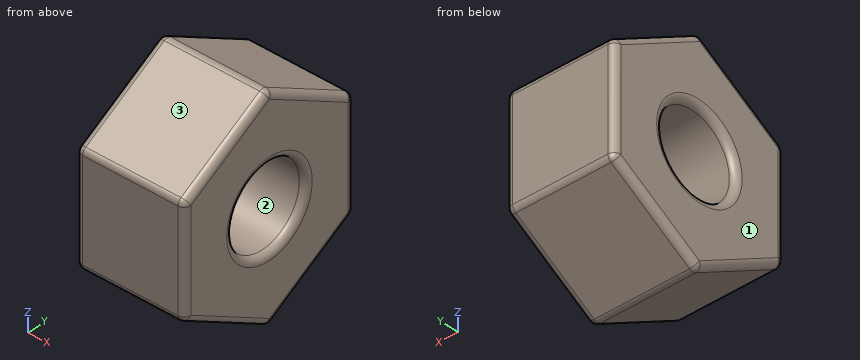
```python
from build123d import *

# Parameters (mm, degrees)
SKETCH1_R           = 3
BOSS_EXTRUDE1_DEPTH = 8
FILLET1_R           = 0.5


with BuildPart() as part:
    # Sketch1 → Boss-Extrude1 (new body)
    with BuildSketch(Plane.YZ):
        Polygon((-6.92820323, -4), (0, -8), (6.92820323, -4), (6.92820323, 4), (0, 8), (-6.92820323, 4), align=None)
        with Locations(Location((0, 0, 0), (0, 0, 270))):
            Circle(SKETCH1_R, mode=Mode.SUBTRACT)
    extrude(amount=BOSS_EXTRUDE1_DEPTH)

    # Fillet1
    fillet1_edges = [part.edges().sort_by_distance(p)[0] for p in [
        (4, -6.92820323, 4),
        (4, 0, 8),
        (4, 6.92820323, 4),
        (4, 6.92820323, -4),
        (4, 0, -8),
        (4, -6.92820323, -4),
        (8, 3.464101615, -6),
        (8, 6.92820323, 0),
        (0, 0, 3),
        (8, 0, 3),
        (8, 3.464101615, 6),
        (8, -3.464101615, 6),
        (8, -6.92820323, 0),
        (0, -3.464101615, 6),
        (0, 3.464101615, 6),
        (0, 6.92820323, 0),
        (0, 3.464101615, -6),
        (0, -3.464101615, -6),
        (0, -6.92820323, 0),
        (8, -3.464101615, -6),
    ]]
    fillet(fillet1_edges, radius=FILLET1_R)


solid = part.part
```
Design review of the part built by this model. Coordinates are the model's own, in mm. Face numbers are marked on the shaded views. Round coordinates to 2 decimals unless told otherwise and drop trailing zeros. Write each loop counter-clockwise with the first axis right and the second up, starting at its lowest first coordinate (ties: lowest second). Pieces come first, ordered by that corner, then holes. Notation, with made-up numbers: (-36, 8.25) -> (20, 8.25) arc R23 ccw to (20, 20.25) -> close; hole circle Ø11 at (62.25, 26.5). An arc over 180 degrees is marked (long way). Answer in a Markdown table with one row per item.
Q1. Clearance check with flat-ended pins moving along their axes: pin 1 Ø1 at (x, y) = (6.5, -1) entering from +Z; pin 2 Ø3 at (x, y) = (6.5, -5) entering from -Z; pin 3 Ø2 at (x, y) = (6.5, -4) entering from -Z; pin 4 Ø3.5 at (y, z) = (0, 0) entering from -X. State where each tip first meets the part, or that it passes through.
The answers:
| item | result |
|---|---|
| pin 1 | z = 7.71 |
| pin 2 | z = -5.98 |
| pin 3 | z = -6.27 |
| pin 4 | through |
Q2. To check wall thickness, follow L1, parallel to Y at x = 5.25, z = 0; L2, parallel to Z at x = 4, y = -1; L3, parallel to Z at x = 4, y = 1.5. State the ranges of each line that lie inside material, in increasing order. Write a range as [from, to].
The answers:
| item | result |
|---|---|
| L1 | [-6.93, -3], [3, 6.93] |
| L2 | [-7.42, -2.83], [2.83, 7.42] |
| L3 | [-7.13, -2.6], [2.6, 7.13] |
Q3. Take a section at A-A, the plane z = 0. State the section outline as (x, y) points.
The answers:
| item | result |
|---|---|
| outline | (0, -6.43) arc R0.5 ccw to (0.5, -6.93) -> (7.5, -6.93) arc R0.5 ccw to (8, -6.43) -> (8, -3.5) arc R0.5 ccw to (7.5, -3) -> (0.5, -3) arc R0.5 ccw to (0, -3.5) -> close; (0, 3.5) arc R0.5 ccw to (0.5, 3) -> (7.5, 3) arc R0.5 ccw to (8, 3.5) -> (8, 6.43) arc R0.5 ccw to (7.5, 6.93) -> (0.5, 6.93) arc R0.5 ccw to (0, 6.43) -> close |
Q4. Take a section at B-B, the plane x = 6. State the section outline as (y, z) points, then the cut area to 3 significant figures.
The answers:
| item | result |
|---|---|
| outline | (-6.93, -3.71) arc R0.5 ccw to (-6.68, -4.14) -> (-0.25, -7.86) arc R0.5 ccw to (0.25, -7.86) -> (6.68, -4.14) arc R0.5 ccw to (6.93, -3.71) -> (6.93, 3.71) arc R0.5 ccw to (6.68, 4.14) -> (0.25, 7.86) arc R0.5 ccw to (-0.25, 7.86) -> (-6.68, 4.14) arc R0.5 ccw to (-6.93, 3.71) -> close; hole circle Ø6 at (0, 0) |
| area | 138 mm² |
Q5. Take a section at C-C, the plane x = 7.75. State the section outline as (y, z) points, then the cut area to 3 significant figures.
The answers:
| item | result |
|---|---|
| outline | (-6.86, -3.71) arc R0.43 ccw to (-6.64, -4.09) -> (-0.22, -7.8) arc R0.43 ccw to (0.22, -7.8) -> (6.64, -4.09) arc R0.43 ccw to (6.86, -3.71) -> (6.86, 3.71) arc R0.43 ccw to (6.64, 4.09) -> (0.22, 7.8) arc R0.43 ccw to (-0.22, 7.8) -> (-6.64, 4.09) arc R0.43 ccw to (-6.86, 3.71) -> close; hole circle Ø6.13 at (0, 0) |
| area | 133 mm² |
Q6. Draft analysis for pull direction Z (two halves, no side actions). For the marked faces 1, 2 and 3, state which applies: +Z half, -Z half, draft (parallel to the pull), parting line (faces both ways), or undercut.
The answers:
| item | result |
|---|---|
| face 1 | draft |
| face 2 | undercut |
| face 3 | +Z half |
